Read the model definition and answer for the solid it produces. Units are mm, in the model's axes. A direction names the side the tool comes from. Coordinates: 2 decimals unless noted, no trailing zeros. Write each loop counter-clockwise with the first axis right and the second up, starting at its lowest first coordinate (ties: lowest second). Pieces come first, ordered by that corner, then holes. Notation, with made-up numbers: (22.5, 9) -> (77.5, 9) arc R15 ccw to (77.5, 29) -> close; hole circle Ø11 at (-38, 50.5). An arc over 180 degrees is marked (long way). Return JSON: item names as keys, results as strings.
from build123d import *

# Parameters (mm, degrees)
BOSS_EXTRUDE1_DEPTH = 25.4
BOSS_EXTRUDE2_DEPTH = 1.27
CIRPATTERN3_COUNT   = 3
SKETCH3_R           = 19.05
BOSS_EXTRUDE3_DEPTH = 5.08


with BuildPart() as part:
    # Sketch1 → Boss-Extrude1 (new body)
    with BuildSketch(Plane(origin=(0, 0, 0), x_dir=(1, 0, 0), z_dir=(0, 1, 0))):
        Polygon((-1.27, 0), (0, 2.199704526), (1.27, 0), align=None)
    extrude(amount=BOSS_EXTRUDE1_DEPTH)

    # Sketch2 → Boss-Extrude2 (add, symmetric)
    with BuildSketch(Plane(origin=(0, 0, 0), x_dir=(0, 0, -1), z_dir=(1, 0, 0))):
        Polygon((0, 0), (-172.909241249, 41.415387125), (-172.909241249, 66.815387125), (0, 25.4), align=None)
    boss_extrude2 = extrude(amount=BOSS_EXTRUDE2_DEPTH, both=True)

    # CirPattern3: Boss-Extrude2 ×3 about axis
    cirpattern3_axis = Axis((0, 0, -0.733234842), (0, 1, 0))
    for i in range(1, CIRPATTERN3_COUNT):
        add(boss_extrude2.rotate(cirpattern3_axis, i * 360 / CIRPATTERN3_COUNT))

    # Sketch3 → Boss-Extrude3 (add)
    with BuildSketch(Plane(origin=(0, 25.4, 0), x_dir=(1, 0, 0), z_dir=(0, 1, 0))):
        Circle(SKETCH3_R)
    extrude(amount=BOSS_EXTRUDE3_DEPTH)


solid = part.part
1. Consider L1, parallel to X at y = 28, z = 49; L2, parallel to X at y = 32.5, z = -60.5; L3, parallel to Z at x = 136.5, y = 45. Determine where each line is inside the solid, lowest interval first.
Taken from the geometry:
{"L1": "x = -1.27 to 1.27", "L2": "x = -106.06 to -100.98, 100.98 to 106.06", "L3": "z = -81.01 to -78.08"}
2. The part is cut by section C-C (y = 7). Determine the outline of the cut face in (x, z) (1 decimal).
Taken from the geometry:
{"outline": "(-26.6, -14.6) -> (-25.3, -16.8) -> (0, -2.2) -> (25.3, -16.8) -> (26.6, -14.6) -> (1.3, 0) -> (1.3, 29.2) -> (-1.3, 29.2) -> (-1.3, 0) -> close"}
3. Flat-ended cylindrical pins translate along their axes: pin 1 Ø4 at (x, y) = (78.5, 36.5) entering from +Z; pin 2 Ø14 at (x, z) = (-7, 6) entering from -Y; pin 3 Ø18.5 at (x, z) = (-0.5, -13.5) entering from -Y. Find the tip coordinate at first contact, or state that the pin passes through.
Taken from the geometry:
{"pin 1": "stops at z = -43.43", "pin 2": "stops at y = 0.47", "pin 3": "stops at y = 25.4"}
4. For a pull along X with two mould halves and no side action, classify faces 1 (the face through (84.169, 48.506, -49.349)), 2 (the face through (-10, 25.4, 5)), 3 (the face through (74.45, 20.42, -43.74)), 4 (the face through (-15.12, 27.9, 11.59)) as +X half, -X half, draft (parallel to the pull), parting line (faces both ways), or undercut.
Taken from the geometry:
{"face 1": "undercut", "face 2": "draft", "face 3": "+X half", "face 4": "undercut"}
5. The part is cut by section D-D (x = 52). Determine the outline of the cut face in (y, z).
Taken from the geometry:
{"outline": "(14.03, -29.29) -> (14.38, -32.22) -> (39.78, -32.22) -> (39.43, -29.29) -> close"}
6. The part is cut by section A-A (y = 36.5). Determine the outline of the cut face in (x, z), then the cut area to 3 significant figures.
Taken from the geometry:
{"outline": "(-133.24, -76.19) -> (-131.97, -78.39) -> (-40.13, -25.37) -> (-41.4, -23.17) -> close; (-1.27, 46.34) -> (1.27, 46.34) -> (1.27, 152.39) -> (-1.27, 152.39) -> close; (40.13, -25.37) -> (131.97, -78.39) -> (133.24, -76.19) -> (41.4, -23.17) -> close", "area": "808 mm2"}
7. The part is cut by section B-B (z = -28). Determine the outline of the cut face in (x, y), then the cut area to 3 significant figures.
Taken from the geometry:
{"outline": "(-49.77, 13.41) -> (-44.69, 12.36) -> (-44.69, 37.76) -> (-49.77, 38.81) -> close; (44.69, 12.36) -> (49.77, 13.41) -> (49.77, 38.81) -> (44.69, 37.76) -> close", "area": "258 mm2"}
8. A tool of negligible diameter and unlimited length cuts with its end or side. For faces 5 (the face through (10, 25.4, 5)), 6 (the face through (0.018, 20.418, 85.244)), 7 (the face through (0, 30.48, 0)), 8 (the face through (0, 25.4, -11)), 9 (the face through (-74.47, 20.42, -43.71)), from which of +Z, -Z, +X, -X, +Y, -Y can it reach the whole face along a straight path? Write none if from no direction.
Taken from the geometry:
{"face 5": "+Z, +X, -Y", "face 6": "+Z, +X, -X, -Y", "face 7": "-Z, +Y", "face 8": "-Z, -Y", "face 9": "-Z, -X, -Y"}
